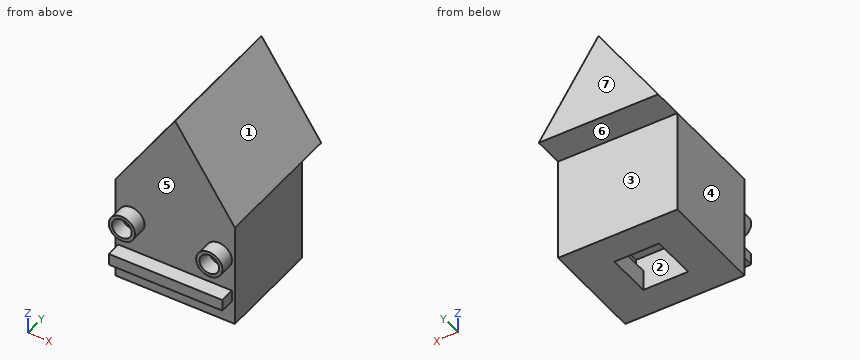
```python
from build123d import *

# Parameters (mm, degrees)
F0_W     = 40
F0_H     = 35
F1_DEPTH = 17.5
F2_W     = 15
F2_H     = 10
F3_DEPTH = 7.5
F4_R     = 4.3956172523
F4_R_2   = 3.2967313173
F4_W     = 38.0061380565
F4_H     = 3.8650305942
F5_DEPTH = 5
F9_DEPTH = 45


# Not quite as in the source:
# - the program builds the solid bodies; features that only make, move or delete a surface that nothing else refers to are left out


with BuildPart() as f1:
    # F0 (on Front) → F1 (new body, symmetric)
    with BuildSketch(Plane.XZ):
        Rectangle(F0_W, F0_H)
    extrude(amount=F1_DEPTH, both=True)

    # F2 (on Front) → F3 (cut, symmetric)
    with BuildSketch(Plane.XZ):
        with Locations((0, -15.5)):
            Rectangle(F2_W, F2_H)
        Polygon((-7.5, -10.5), (7.5, -10.5), (10, -10.5), (10, -5.5), (-10, -5.5), (-10, -10.5), align=None)
    extrude(amount=F3_DEPTH, both=True, mode=Mode.SUBTRACT)

    # F4 (on face) → F5 (join)
    with BuildSketch(Plane.XZ.offset(17.5)):
        with Locations((-14.6328676492, 5.2709789015)):
            Circle(F4_R)
        with Locations((-14.6328676492, 5.2709789015)):
            Circle(F4_R_2, mode=Mode.SUBTRACT)
        with Locations((14.6328676492, 5.2709789015)):
            Circle(F4_R)
        with Locations((14.6328676492, 5.2709789015)):
            Circle(F4_R_2, mode=Mode.SUBTRACT)
        with Locations((0, -7.730061654)):
            Rectangle(F4_W, F4_H)
    extrude(amount=F5_DEPTH)

    # F4 (on face) → F9 (join)
    with BuildSketch(Plane.XZ.offset(17.5)):
        Polygon((0, 47.5069768727), (-20, 17.5), (20, 17.5), align=None)
    extrude(amount=-F9_DEPTH)


solid = f1.part
```
Input: part model. Units: mm. Frame: model coordinates. Face numbers are marked on the shaded views. A direction names the side the tool comes from. Round coordinates to 2 decimals unless told otherwise and drop trailing zeros. Loops run counter-clockwise (first coordinate to the right, second up) from the corner with the lowest first, then second, coordinate; pieces in that order, holes last. Notation, with made-up numbers: M -40,12 L -4,12 A19 cw -4,29 Z; hole C -19,41 d7. An arc over 180 degrees is marked long. Answer in a Markdown table with one row per item. Add a question column.
1. Section D-D (x = 9). Output: boundary loops of the cut face in (y, z).
2. Ray query, probe 1 along X at (y, z) = (-18.5, 5.5); probe 2 along X at (y, z) = (5, -8); probe 3 along Y at (x, z) = (12, 22). Return the intervals inside material, ascending.
3. Mould query, pull axis X, two halves, no side actions, for the marked faces 1, 2, 3 and 4. Classes: released by +X, released by -X, zero draft, split by the parting line, or undercut.
4. Set-up query: the marked faces 5, 6 and 7. Return all of +Z, -Z, +X, -X, +Y, -Y with unobstructed straight access to the full face (end or side cutting, diameter ignored); none if empty.
5. Section A-A (y = -6). Output: boundary loops of the cut face in (x, z), and give its area (3 significant figures).
6. Section B-B (z = 7.5). Output: boundary loops of the cut face in (x, y), and give its area (3 significant figures).
7. Contact query for flat-ended pins moving along their axis: pin 1 (2 mm diameter, centred on y = 18.5, z = 22, fed in from -X); pin 2 (7.5 mm diameter, centred on x = 14.63, z = 5.27, fed in from -Y); pin 3 (3.5 mm diameter, centred on x = 14.5, z = 5.5, fed in from -Y); pin 4 (8 mm diameter, centred on y = 6.5, z = 23.5, fed in from +X). Output: stop coordinate, or through.
8. Section C-C (x = 5). Output: boundary loops of the cut face in (y, z).
Values follow:
| question | item | result |
|---|---|---|
| 1 | outline | M -22.5,-9.66 L -17.5,-9.66 L -17.5,-17.5 L 17.5,-17.5 L 17.5,17.5 L 27.5,17.5 L 27.5,34 L -17.5,34 L -17.5,-5.8 L -22.5,-5.8 Z; hole M -7.5,-10.5 L 7.5,-10.5 L 7.5,-5.5 L -7.5,-5.5 Z |
| 2 | probe 1 | -19.02 to -17.92, -11.34 to -10.24, 10.24 to 11.34, 17.92 to 19.02 |
| 2 | probe 2 | -20 to -10, 10 to 20 |
| 2 | probe 3 | -17.5 to 27.5 |
| 3 | face 1 | released by +X |
| 3 | face 2 | undercut |
| 3 | face 3 | zero draft |
| 3 | face 4 | released by -X |
| 4 | face 5 | -Y |
| 4 | face 6 | -Z, +X, -X, +Y |
| 4 | face 7 | +Z, -Z, +X, -X, +Y |
| 5 | outline | M -20,-17.5 L -7.5,-17.5 L -7.5,-10.5 L -10,-10.5 L -10,-5.5 L 10,-5.5 L 10,-10.5 L 7.5,-10.5 L 7.5,-17.5 L 20,-17.5 L 20,17.5 L 0,47.51 L -20,17.5 Z |
| 5 | area | 1,800 mm^2 |
| 6 | outline | M -20,-17.5 L -18.42,-17.5 L -18.42,-22.5 L -17.06,-22.5 L -17.06,-17.5 L -12.2,-17.5 L -12.2,-22.5 L -10.84,-22.5 L -10.84,-17.5 L 10.84,-17.5 L 10.84,-22.5 L 12.2,-22.5 L 12.2,-17.5 L 17.06,-17.5 L 17.06,-22.5 L 18.42,-22.5 L 18.42,-17.5 L 20,-17.5 L 20,17.5 L -20,17.5 Z |
| 6 | area | 1,430 mm^2 |
| 7 | pin 1 | x = -17.67 |
| 7 | pin 2 | y = -22.5 |
| 7 | pin 3 | y = -17.5 |
| 7 | pin 4 | x = 18.67 |
| 8 | outline | M -22.5,-9.66 L -17.5,-9.66 L -17.5,-17.5 L -7.5,-17.5 L -7.5,-5.5 L 7.5,-5.5 L 7.5,-17.5 L 17.5,-17.5 L 17.5,17.5 L 27.5,17.5 L 27.5,40.01 L -17.5,40.01 L -17.5,-5.8 L -22.5,-5.8 Z |
